Verification items for the finished model (mm, model axes). A direction names the side the tool comes from. Coordinates: 2 decimals unless noted, no trailing zeros. Loops run counter-clockwise (first coordinate to the right, second up) from the corner with the lowest first, then second, coordinate; pieces in that order, holes last. Notation, with made-up numbers: (65, -4) - (69, -4) arc R17 cw to (69, 18) - close; hole circle Ø3 at (43, 28.5). An arc over 180 degrees is marked (long way). Answer as CSV lines item,"result". Start each with the question number.
1. Material ranges on line 1 (Y direction, x = 131, z = 58.5); line 2 (Z direction, x = 62, y = 7); line 3 (X direction, y = 4, z = 8), recorded low to high. Write a range as [from, to].
2. Cross-section at C-C (z = 68). Enter the section's corners in (x, y), plus the area to 3 significant figures.
3. Cross-section at D-D (z = 139). Enter the section's corners in (x, y).
4. Cross-section at B-B (x = 19.5). Enter the section's corners in (y, z), plus the area to 3 significant figures.
5. Set-up check for faces 1 (the cylindrical face through (108.54, 8.04, 110.95)), 2 (the cylindrical face through (92.04, 8.02, 94.09)), 3 (the cylindrical face through (110.383, 22.122, 107.982)): record each of +Z, -Z, +X, -X, +Y, -Y from which the full face is reachable in a straight line by a thin tool's end or side.
6. Cross-section at A-A (y = 5.5). Enter the section's corners in (x, z), plus the area to 3 significant figures.
7. Release check for a two-part mould opening along X. For faces 4 (the flat face through (0, 0.5, 143.6)), 5 (the flat face through (100, 14.274, 85)), 6 (the cylindrical face through (109.816, 14.886, 107.427)) record: pulls with the +X half, pulls with the -X half, needs draft (parallel to the pull), parting line crosses it, or undercut.
8. Gauge pin test, flat ends, axial feed: P1, Ø8, axis at y = 3.5, z = 74.5, coming from the -X side; P2, Ø8, axis at y = 10, z = 43, coming from the -X side; P3, Ø12, axis at y = 23.5, z = 66, coming from the +X side; P4, Ø6, axis at x = 111, z = 105, coming from the -Y side. Record the tip position at first contact, or that the pin passes through.
Autodesk Inventor part; units mm, degrees
ref_plane "YZ Plane" through (0, 0, 0) normal (1, 0, 0) x (0, 1, 0)
ref_plane "XZ Plane" through (0, 0, 0) normal (0, 1, 0) x (-1, 0, 0)
ref_plane "XY Plane" through (0, 0, 0) normal (0, 0, 1) x (1, 0, 0)
sketch "Sketch1" plane through (0, 0, 0) normal (1, 0, 0) x (0, 1, 0)
  line L0 (0, 0) -> (73.993, 0)
  line L1 (0, 130.0359) -> (44.4227, 130.0359)
  line L2 (0, 130.0359) -> (0, 155.2107)
  line L3 (0, 155.2107) -> (15.8613, 155.2107)
  line L4 (44.4227, 155.2107) -> (44.4227, 130.0359)
  line L5 (28.5613, 153.6232) -> (1.5875, 153.6232)
  line L6 (1.5875, 153.6232) -> (1.5875, 131.6234)
  line L7 (1.5875, 131.6234) -> (42.8352, 131.6234)
  line L8 (42.8352, 131.6234) -> (42.8352, 153.6232)
  line L9 (18.2426, 143.1015) -> (18.2426, 119.3292)
  line L10 (14.2738, 131.6234) -> (14.2738, 130.0359)
  line L11 (22.2113, 131.6234) -> (22.2113, 130.0359)
  line L12 (22.2113, 154.417) -> (28.5613, 154.417)
  line L13 (28.5613, 154.417) -> (28.5613, 153.6232)
  line L14 (22.2113, 154.417) -> (15.8613, 154.417)
  line L15 (15.8613, 154.417) -> (15.8613, 155.2107)
  line L16 (22.2113, 172.7158) -> (22.2113, 154.417)
  line L17 (22.2113, 153.6232) -> (22.2113, 148.8604)
  dimension "d1" = 25.1748
  dimension "d2" = 130.0359
  dimension "Height" = 44.4227
  dimension "d4" = 0
  dimension "d5" = 1.5875
  dimension "d6" = 1.5875
  dimension "d7" = 1.5875
  dimension "d8" = 1.5875
  dimension "d9" = 18.2426
  dimension "d10" = 7.9375
  dimension "d11" = 3.9688
  dimension "d14" = 0.7937
  dimension "d15" = 6.35
  dimension "d16" = 6.35
revolve "Revolution1" add sketch "Sketch1" angle 90 about axis through (0, 0, 0) along (0, 1, 0) contours L2 L3 L15 L14 L12 L13 L5 L6 L7 L10 L1
equation "\"d2\" = 0.5 * IBDia - 3 * SpWall"
equation "\"Height\" = Wall + 4 * SpWall + BevDriverDia + d1_1"
equation "\"d5\" = Wall"
equation "\"d6\" = Wall"
equation "\"d7\" = Wall"
equation "\"d8\" = Wall"
equation "\"d9\" = 2 * SpWall + 0.5 * BevDriverDia"
equation "\"d10\" = AxelDia + Space"
equation "\"d11\" = 0.5 * Space + 0.5 * AxelDia"
equation "\"d14\" = 0.5 * Wall"
equation "\"IDia\" = 266.7"
equation "\"Wall\" = 1.5875"
equation "\"Space\" = 1.5875"
equation "\"SpWall\" = 3.175"
equation "\"AxelDia\" = 6.35"
equation "\"d13\" = 0.5 * Height"
properties part number "OuterShell_Bottom_Quarter"
Values follow:
1,line 1,"y = [0, 1.59]"
1,line 2,"z = [114.3, 116.11], [140.56, 142.29]"
1,line 3,"x = [129.79, 131.38], [153.41, 155]"
2,outline,"(110.84, 0) - (139.52, 0) - (139.52, 15.86) - (138.64, 15.86) - (138.64, 28.56) - (137.75, 28.56) - (137.75, 1.59) - (112.7, 1.59) - (112.7, 14.27) - (110.84, 14.27) - close"
2,area,"106 mm²"
3,outline,"(0, 0) - (69.06, 0) - (69.06, 15.86) - (67.26, 15.86) - (67.26, 28.56) - (65.41, 28.56) - (65.41, 1.59) - (0, 1.59) - close"
4,outline,"(0, 128.57) - (14.27, 128.57) - (14.27, 130.17) - (1.59, 130.17) - (1.59, 152.38) - (28.56, 152.38) - (28.56, 153.18) - (15.86, 153.18) - (15.86, 153.98) - (0, 153.98) - close"
4,area,"93.7 mm²"
5,face 1,"+Z, +X, +Y, -Y"
5,face 2,"+Y"
5,face 3,"+Z, +X, +Y"
6,outline,"(0, 130.04) arc R130.04 cw to (130.04, 0) - (131.62, 0) arc R131.62 ccw to (0, 131.62) - close; (0, 153.62) arc R153.62 cw to (153.62, 0) - (155.21, 0) arc R155.21 ccw to (0, 155.21) - close"
6,area,"711 mm²"
7,face 4,"pulls with the -X half"
7,face 5,"needs draft"
7,face 6,"undercut"
8,P1,"stops at x = 103.67"
8,P2,"stops at x = 121.24"
8,P3,"stops at x = 142.28"
8,P4,"stops at y = 0"
